from build123d import *

# Parameters (mm, degrees)
F1_START      = -1
F0_W          = 16
F0_H          = 2.4
F0_W_2        = 2.4
F0_H_2        = 16
F1_DEPTH      = 2.4
F0_W_3        = 31.3
F0_H_3        = 33.8
F2_DEPTH      = 2
F2_DEPTH_BACK = 3.4
F4_W          = 28.1
F4_H          = 30.6
F4_W_2        = 26.5
F4_H_2        = 29
F5_DEPTH      = 2.3
F6_START      = 1.2
F3_W          = 0.8
F3_H          = 4
F3_W_2        = 0.2
F3_W_3        = 0.5
F6_DEPTH      = 0.8
F7_START      = 2
F7_DEPTH      = 2.3
F8_START      = 3.2
F8_DEPTH      = 1.1
F9_R          = 0.5
F11_START     = 14
F10_W         = 17
F10_H         = 7
F11_DEPTH     = 4
F12_R         = 1.5
F14_SIZE      = 0.8


# Not quite as in the source:
# - a feature names something its author has since deleted; it is built from what else it names


with BuildPart() as f1:
    # F0 (on Top) → F1 (new body)
    with BuildSketch(Plane.XY.offset(F1_START)):
        Polygon((-8, 14.5), (-13.25, 14.5), (-13.25, 8), (-10.85, 8), (-10.85, -8), (-13.25, -8), (-13.25, -14.5), (-8, -14.5), (-8, -12.1), (8, -12.1), (8, -14.5), (13.25, -14.5), (13.25, -8), (10.85, -8), (10.85, 8), (13.25, 8), (13.25, 14.5), (8, 14.5), (8, 12.1), (-8, 12.1), align=None)
        with Locations((0, -13.3)):
            Rectangle(F0_W, F0_H)
        with Locations((-12.05, 0)):
            Rectangle(F0_W_2, F0_H_2)
        with Locations((12.05, 0)):
            Rectangle(F0_W_2, F0_H_2)
        with Locations((0, 13.3)):
            Rectangle(F0_W, F0_H)
    extrude(amount=-F1_DEPTH)

    # F0 (on Top) → F2 (join, two sides)
    with BuildSketch(Plane.XY) as f2_sk:
        Rectangle(F0_W_3, F0_H_3)
        Polygon((-13.25, 8), (-13.25, 14.5), (-8, 14.5), (8, 14.5), (13.25, 14.5), (13.25, 8), (13.25, -8), (13.25, -14.5), (8, -14.5), (-8, -14.5), (-13.25, -14.5), (-13.25, -8), align=None, mode=Mode.SUBTRACT)
    extrude(amount=F2_DEPTH)
    extrude(f2_sk.sketch, amount=-F2_DEPTH_BACK)

    # F4 (on face) → F5 (join)
    with BuildSketch(Plane.XY.offset(2)):
        Rectangle(F4_W, F4_H)
        Rectangle(F4_W_2, F4_H_2, mode=Mode.SUBTRACT)
    extrude(amount=F5_DEPTH)

    # F3 (on Top) → F6 (join)
    with BuildSketch(Plane.XY.offset(F6_START)):
        with Locations((-13.6500000894, 6.5681297779)):
            Rectangle(F3_W, F3_H)
        with Locations((-14.1500000894, 6.5681297779)):
            Rectangle(F3_W_2, F3_H)
        with Locations((-14.5000000894, 6.5681297779)):
            Rectangle(F3_W_3, F3_H)
        with Locations((13.6499995038, 6.5681299639)):
            Rectangle(F3_W, F3_H)
        with Locations((14.1499995038, 6.5681299639)):
            Rectangle(F3_W_2, F3_H)
        with Locations((14.4999995038, 6.5681299639)):
            Rectangle(F3_W_3, F3_H)
        with Locations((-14.1500000894, -6.5681295022)):
            Rectangle(F3_W_2, F3_H)
        with Locations((-14.5000000894, -6.5681295022)):
            Rectangle(F3_W_3, F3_H)
        with Locations((-13.6500000894, -6.5681295022)):
            Rectangle(F3_W, F3_H)
        with Locations((14.1499995038, -6.5681295022)):
            Rectangle(F3_W_2, F3_H)
        with Locations((14.4999995038, -6.5681295022)):
            Rectangle(F3_W_3, F3_H)
        with Locations((13.6499995038, -6.5681295022)):
            Rectangle(F3_W, F3_H)
    extrude(amount=F6_DEPTH)

    # F3 (on Top) → F7 (join)
    with BuildSketch(Plane.XY.offset(F7_START)):
        with Locations((-13.6500000894, -6.5681295022)):
            Rectangle(F3_W, F3_H)
        with Locations((-13.6500000894, 6.5681297779)):
            Rectangle(F3_W, F3_H)
        with Locations((13.6499995038, -6.5681295022)):
            Rectangle(F3_W, F3_H)
        with Locations((13.6499995038, 6.5681299639)):
            Rectangle(F3_W, F3_H)
    extrude(amount=F7_DEPTH)

    # F3 (on Top) → F8 (join)
    with BuildSketch(Plane.XY.offset(F8_START)):
        with Locations((-14.5000000894, 6.5681297779)):
            Rectangle(F3_W_3, F3_H)
        with Locations((-14.1500000894, 6.5681297779)):
            Rectangle(F3_W_2, F3_H)
        with Locations((-14.5000000894, -6.5681295022)):
            Rectangle(F3_W_3, F3_H)
        with Locations((-14.1500000894, -6.5681295022)):
            Rectangle(F3_W_2, F3_H)
        with Locations((14.4999995038, 6.5681299639)):
            Rectangle(F3_W_3, F3_H)
        with Locations((14.1499995038, 6.5681299639)):
            Rectangle(F3_W_2, F3_H)
        with Locations((14.4999995038, -6.5681295022)):
            Rectangle(F3_W_3, F3_H)
        with Locations((14.1499995038, -6.5681295022)):
            Rectangle(F3_W_2, F3_H)
    extrude(amount=F8_DEPTH)

    # F9
    f9_edges = [f1.edges().sort_by_distance(p)[0] for p in [
        (13.25, 6.56813, 1.2),
        (14.75, 6.56813, 3.2),
        (-14.75, 6.56813, 3.2),
        (-14.75, 6.56813, 4.3),
        (14.75, -6.56813, 4.3),
        (14.75, -6.56813, 3.2),
        (13.25, -6.56813, 1.2),
        (-14.75, -6.56813, 4.3),
        (-14.75, -6.56813, 3.2),
        (14.75, 6.56813, 4.3),
    ]]
    fillet(f9_edges, radius=F9_R)

    # F10 (on Front) → F11 (cut)
    with BuildSketch(Plane.XZ.offset(F11_START)):
        with Locations((-4.619e-07, 2.5000009835)):
            Rectangle(F10_W, F10_H)
    extrude(amount=F11_DEPTH, mode=Mode.SUBTRACT)

    # F12
    f12_edges = [f1.edges().sort_by_distance(p)[0] for p in [
        (15.65, -16.9, -0.7),
        (15.65, 16.9, -0.7),
        (-15.65, 16.9, -0.7),
        (-15.65, -16.9, -0.7),
    ]]
    fillet(f12_edges, radius=F12_R)

    # F14
    f14_edges = [f1.edges().sort_by_distance(p)[0] for p in [
        (-14.05, 15.3, 3.15),
        (14.05, 15.3, 3.15),
        (-14.05, -15.3, 3.15),
        (14.05, -15.3, 3.15),
    ]]
    chamfer(f14_edges, length=F14_SIZE)


solid = f1.part
Can you work these out from the model? Positions are in its coordinate system, mm. A direction names the side the tool comes from. Coordinates: 2 decimals unless noted, no trailing zeros. Write each loop counter-clockwise with the first axis right and the second up, starting at its lowest first coordinate (ties: lowest second). Pieces come first, ordered by that corner, then holes. Notation, with made-up numbers: (58.25, 34) -> (102.25, 34) arc R10 ccw to (102.25, 48) -> close; hole circle Ø10 at (11.5, 77.5). An arc over 180 degrees is marked (long way). Write each question's results on one line, items separated by ' | '. Start each with the question number.
Q1. On a 3-axis mill with a long thin cutter (end or side, diameter ignored), from which of +Z, -Z, +X, -X, +Y, -Y can I reach the whole of each face in a straight line? I mean faces 4 (the face through (8.5, -15, 1)), 5 (the face through (-11, -15.3, 3)), 6 (the face through (0, 16.9, -1)), 7 (the face through (13.64, 14.91, 3.13)), 8 (the face through (0, 14.5, 2)). Say none if no direction works.
Q2. If I drill on probe 1 along X at (y, z) = (-13, 3.5); probe 2 along Y at (x, z) = (-12.5, 2.5); probe 3 along X at (y, z) = (12.5, 1.5), over which ranges is the centre line in solid material (lowest first)?
Q3. Imagine slicing it at C-C (y = 4). Write out the boundary of the cut face in (x, z), then the cut area to 3 significant figures.
Q4. Imagine slicing it at D-D (z = 0.25). Write out the boundary of the cut face in (x, y), then the cut area to 3 significant figures.
Q5. We'd pull the mould along Y, two halves only. Please class faces 1 (the face through (0, 0, -1)), 2 (the face through (-15.22, 16.45, -0.74)), 3 (the face through (13.66, -14.89, 3.13)): +Y half, -Y half, draft (parallel to the pull), parting line (faces both ways), or undercut.
Q6. I'm going to push flat-ended pins straight in: pin 1 (1.2 mm diameter, centred on y = -2, z = 3.5, fed in from +X); pin 2 (2.5 mm diameter, centred on y = -16, z = 2, fed in from +X); pin 3 (0.8 mm diameter, centred on x = 14.5, z = 4, fed in from -Y); pin 4 (1.2 mm diameter, centred on x = 11.5, z = 3.5, fed in from -Y). Where does each tip first touch, or does it pass through?
Q7. Imagine slicing it at A-A (z = 2.75). Write out the boundary of the cut face in (x, y).
Taken from the geometry:
1) face 4: +Z, -Y | face 5: +Z, +X, -X, -Y | face 6: +Z, -Z, +X, -X, +Y | face 7: +Z, +X, +Y | face 8: +Z
2) probe 1: x = -14.05 to -13.25, 13.25 to 14.05 | probe 2: y = -15.3 to -14.5, 14.5 to 15.3 | probe 3: x = -15.65 to -13.25, 13.25 to 15.65
3) outline: (-15.65, -3.4) -> (15.65, -3.4) -> (15.65, 2) -> (14.05, 2) -> (14.05, 4.3) -> (13.25, 4.3) -> (13.25, -1) -> (-13.25, -1) -> (-13.25, 4.3) -> (-14.05, 4.3) -> (-14.05, 2) -> (-15.65, 2) -> close | area: 93.2 mm^2
4) outline: (-15.65, -15.4) arc R1.5 ccw to (-14.15, -16.9) -> (-8.5, -16.9) -> (-8.5, -14.5) -> (-13.25, -14.5) -> (-13.25, 14.5) -> (13.25, 14.5) -> (13.25, -14.5) -> (8.5, -14.5) -> (8.5, -16.9) -> (14.15, -16.9) arc R1.5 ccw to (15.65, -15.4) -> (15.65, 15.4) arc R1.5 ccw to (14.15, 16.9) -> (-14.15, 16.9) arc R1.5 ccw to (-15.65, 15.4) -> close | area: 247 mm^2
5) face 1: undercut | face 2: +Y half | face 3: -Y half
6) pin 1: stops at x = 14.05 | pin 2: stops at x = 15.65 | pin 3: stops at y = -8.57 | pin 4: stops at y = -15.3
7) outline: (-14.05, -14.5) -> (-13.25, -15.3) -> (-8.5, -15.3) -> (-8.5, -14.5) -> (-13.25, -14.5) -> (-13.25, 14.5) -> (13.25, 14.5) -> (13.25, -14.5) -> (8.5, -14.5) -> (8.5, -15.3) -> (13.25, -15.3) -> (14.05, -14.5) -> (14.05, 14.5) -> (13.25, 15.3) -> (-13.25, 15.3) -> (-14.05, 14.5) -> close
